Autodesk Inventor part; units mm, degrees
ref_plane "YZ Plane" through (0, 0, 0) normal (1, 0, 0) x (0, 1, 0)
ref_plane "XZ Plane" through (0, 0, 0) normal (0, 1, 0) x (-1, 0, 0)
ref_plane "XY Plane" through (0, 0, 0) normal (0, 0, 1) x (1, 0, 0)
sketch "Sketch1" plane through (0, 0, 0) normal (0, 0, 1) x (1, 0, 0)
  line L0 (0, 94.1479) -> (-14, 94.1843)
  line L1 (0, 0) -> (-14, 0)
  line L2 (-14, 0) -> (-14, 94.1843)
  line L3 (-14, 94.1843) -> (0, 94.1843)
  line L4 (0, 94.1843) -> (0, 0)
  line L5 (-14, 94.1843) -> (0, 94.1843)
  line L6 (0, 94.1843) -> (0, 114.1843)
  line L7 (0, 114.1843) -> (-14, 114.1843)
  line L8 (-14, 114.1843) -> (-14, 94.1843)
  line L9 (0, 0) -> (0, -4)
  line L10 (0, -4) -> (-14, -4)
  line L11 (-14, 0) -> (-14, -4)
  point P0 (0, 88.7812)
  point P1 (0, 94.1479)
  dimension "d0" = 20
  dimension "d7" = 4
extrude "Extrusion1" add sketch "Sketch1" along normal blind 2 contours L4 L1 L2 L0
sketch "Sketch2" plane through (0, 0, 2) normal (0, 0, 1) x (1, 0, 0)
  circle A0 centre (-5.7096, 36.7123) radius 6.15
  circle A1 centre (-5.7096, 36.7123) radius 2.15
  circle A2 centre (-6.8781, 4.5836) radius 17.5
  circle A3 centre (-6.8781, 4.5836) radius 5
  circle A4 centre (-6.8781, 4.5836) radius 32.15
  circle A5 centre (-6.8781, 36.7336) radius 2.25
  line L0 (-6.8781, 4.5836) -> (-6.8781, 17.8952) construction
  line L1 (-6.8781, 36.7336) -> (-6.8781, 4.5836) construction
  line L2 (-11.8781, -0.9531) -> (-11.8781, 14.8638)
  line L3 (-11.8781, 14.8638) -> (-1.8781, 14.8638)
  line L4 (-1.8781, 14.8638) -> (-1.8781, -0.9531)
  line L5 (-1.8781, -0.9531) -> (-11.8781, -0.9531)
  arc A6 (-11.8781, -0.4164) -> (-1.8781, -0.4164) centre (-6.8781, -0.4164) ccw
  point P0 (0, 0)
  point P1 (-1.8781, 4.5836)
  point P2 (-11.8781, 4.5836)
  dimension "d3" = 4.5
  dimension "d4" = 0
extrude "Extrusion2" cut sketch "Sketch2" against normal through all contours A5 A1 A4 | A4 A1 A5 | A4 A5 A1 | A1 A5 A4 | A3 | L4 A6 L5 L2 A3 | A3 L2 L3 L4 | L4 L5 A6 | A6 L5 L2 picked at (-8.3259, 37.2162) picked at (-8.3126, 36.1952) picked at (-6.3657, 36.0685) picked at (-6.3452, 37.3793)
equation "\"BendRadius\" = Thickness"
equation "\"BendReliefWidth\" = Thickness"
equation "\"BendReliefDepth\" = 0.5 * Thickness"
equation "\"CornerReliefSize\" = 4 * Thickness"
equation "\"MinimumRemnant\" = 2 * Thickness"
equation "\"TransitionRadius\" = BendRadius"
equation "\"JacobiRadiusSize\" = BendRadius"
equation "\"GapSize\" = Thickness"
properties part number "backWheelNoMotor brake mount" material "Steel, Mild"
Build history of the part. All positions in model axes, mm. A direction names the side the tool comes from. Round coordinates to 2 decimals unless told otherwise and drop trailing zeros. Write each loop counter-clockwise with the first axis right and the second up, starting at its lowest first coordinate (ties: lowest second). Pieces come first, ordered by that corner, then holes. Notation, with made-up numbers: (21.25, 16.5) - (47.25, 16.5) arc R25 ccw to (47.25, 35.5) - close; hole circle Ø11 at (16.25, 41.5). An arc over 180 degrees is marked (long way). Write each question's results on one line, items separated by ' | '. Start each with the question number.
Item 1: Mould opens along X. For faces 1 (the face through (-7, 14.864, 1)), 2 (the face through (-7, 48, 2)), 3 (the face through (0, 48, 1)) say: pulls with the +X half, pulls with the -X half, needs draft (parallel to the pull), parting line crosses it, or undercut.
Item 2: Saw through at B-B (z = 1.7). Write the cut outline in (x, y).
Item 3: Wall check: L1, parallel to X at y = 8, z = 1.5; L2, parallel to Y at x = -2.25, z = 1.25; L3, parallel to Y at x = -5, z = 0.5. Give the ranges that are in metal, low to high. Write a range as [from, to].
Item 4: Saw through at A-A (x = -7.5). Write the cut outline in (y, z).
Item 5: Drop flat-ended pins along their axis: P1, Ø1, axis at x = -12.5, z = 1.5, coming from the +Y side; P2, Ø3.5, axis at x = -6.88, y = 36.73, coming from the -Z side. Give the stop position or say it passes through.
Item 6: Which spindle directions (+Z, -Z, +X, -X, +Y, -Y) get a long thin tool onto all of the face, cutting with end or side? Do faces 4 (the face through (-11.878, 7, 1)), 5 (the face through (-13, 0, 1)). Say none if no direction does.
Results are:
1) face 1: undercut | face 2: needs draft | face 3: pulls with the +X half
2) outline: (-14, 0) - (-11.88, 0) - (-11.88, 14.86) - (-1.88, 14.86) - (-1.88, 0) - (0, 0) - (0, 94.15) - (-14, 94.18) - close; hole circle Ø4.5 at (-6.88, 36.73)
3) L1: x = [-14, -11.88], [-1.88, 0] | L2: y = [14.86, 94.15] | L3: y = [14.86, 35.49], [37.97, 94.16]
4) outline: (14.86, 0) - (34.57, 0) - (34.57, 2) - (14.86, 2) - close; (38.9, 0) - (94.17, 0) - (94.17, 2) - (38.9, 2) - close
5) P1: stops at y = 94.18 | P2: passes through
6) face 4: +Z, -Z, -Y | face 5: +Z, -Z, +X, -X, -Y
